from build123d import *

# Parameters (mm, degrees)
F0_R     = 12.5
F0_R_2   = 10
F1_DEPTH = 6
F0_R_3   = 2.2
F2_DEPTH = 11
F3_R     = 1.5
F4_DEPTH = 11
F5_DEPTH = 3


with BuildPart() as f1:
    # F0 (on Front) → F1 (new body)
    with BuildSketch(Plane.XZ):
        Circle(F0_R)
        Circle(F0_R_2, mode=Mode.SUBTRACT)
    extrude(amount=F1_DEPTH)

    # F0 (on Front) → F2 (join)
    with BuildSketch(Plane.XZ):
        Circle(F0_R_2)
        Circle(F0_R_3, mode=Mode.SUBTRACT)
    extrude(amount=F2_DEPTH)

    # F3 (on Front) → F4 (cut)
    with BuildSketch(Plane.XZ):
        with Locations((6.3, 0)):
            Circle(F3_R)
        with Locations((-6.3, 0)):
            Circle(F3_R)
    extrude(amount=F4_DEPTH, mode=Mode.SUBTRACT)

    # F3 (on Front) → F5 (cut)
    with BuildSketch(Plane.XZ):
        Polygon((7.970619, 2.845979), (4.670619, 2.869788), (3, 0.023809), (4.629381, -2.845979), (7.929381, -2.869788), (9.6, -0.023809), align=None)
        with Locations((6.3, 0)):
            Circle(F3_R, mode=Mode.SUBTRACT)
        Polygon((-9.6, -0.023809), (-7.929381, -2.869788), (-4.629381, -2.845979), (-3, 0.023809), (-4.670619, 2.869788), (-7.970619, 2.845979), align=None)
        with Locations((-6.3, 0)):
            Circle(F3_R, mode=Mode.SUBTRACT)
    extrude(amount=F5_DEPTH, mode=Mode.SUBTRACT)


solid = f1.part
Input: part model. Units: mm. Frame: model coordinates. A direction names the side the tool comes from. Give positions to 0.01 mm unless a question says otherwise; leave off trailing zeros. Loops run counter-clockwise (first coordinate to the right, second up) from the corner with the lowest first, then second, coordinate; pieces in that order, holes last. Notation, with made-up numbers: (60.5, 58.25) -> (110.5, 58.25) arc R12 ccw to (110.5, 68.25) -> close; hole circle Ø11 at (30, -26). An arc over 180 degrees is marked (long way). Answer as a JSON object with one key per item and string values. Group by question number.
Item 1: Cut plane D-D, the plane x = 9. Return the cut outline in (y, z).
Item 2: Line query: probe 1 along Z at (x, y) = (0, -6.5); probe 2 along Z at (x, y) = (0, -4.5); probe 3 along X at (y, z) = (-8.75, -0.25). Output: solid intervals per line, ascending.
Item 3: Reachability of faces 4 (the flat face through (-2.4, -11, 0.1)), 5 (the flat face through (8.797, -1.479, 1.391)) from +Z, -Z, +X, -X, +Y, -Y: full face, straight path, thin tool, end or side. Return the list, or none.
Item 4: Cut plane C-C, the plane z = -5.75. Return the cut outline in (x, y), and give its area (3 significant figures).
Item 5: Cut plane A-A, the plane x = 0. Return the cut outline in (y, z).
Item 6: Pull-direction query (X, two-part tool) for faces 1 (the flat face through (-0.1, -6, 10.2)), 2 (the cylindrical face through (11.923, -2.958, 3.755)), 3 (the cylindrical face through (-4.87, -6.94, 0.45)); classes: released by +X, released by -X, zero draft, split by the parting line, or undercut.
Item 7: Cut plane B-B, the plane y = -5. Return the cut outline in (x, z).
Item 8: Pin query (flat end, axial travel): P1, Ø1.5, axis at y = -3.5, z = 4.5, coming from the -X side; P2, Ø2, axis at x = 2.5, y = -8.5, coming from the +Z side; P3, Ø4, axis at y = -9, z = -3.5, coming from the +X side. Return the tip coordinate at first contact, or that it passes through.
Checks:
{
 "1": {"outline": "(-11, -4.36) -> (-6, -4.36) -> (-6, -8.67) -> (0, -8.67) -> (0, -1.05) -> (-3, -1.05) -> (-3, 1.03) -> (0, 1.03) -> (0, 8.67) -> (-6, 8.67) -> (-6, 4.36) -> (-11, 4.36) -> close"},
 "2": {"probe 1": "z = -10 to -2.2, 2.2 to 10", "probe 2": "z = -12.5 to -2.2, 2.2 to 12.5", "probe 3": "x = -10 to -7.78, -4.82 to -2.19, 2.19 to 4.82, 7.78 to 10"},
 "3": {"face 4": "+Z, -Z, +X, -X, -Y", "face 5": "+Y"},
 "4": {"outline": "(-11.1, -6) -> (-8.18, -6) -> (-8.18, -11) -> (8.18, -11) -> (8.18, -6) -> (11.1, -6) -> (11.1, 0) -> (-11.1, 0) -> close", "area": "215 mm²"},
 "5": {"outline": "(-11, -10) -> (-6, -10) -> (-6, -12.5) -> (0, -12.5) -> (0, -2.2) -> (-11, -2.2) -> close; (-11, 2.2) -> (0, 2.2) -> (0, 12.5) -> (-6, 12.5) -> (-6, 10) -> (-11, 10) -> close"},
 "6": {"face 1": "zero draft", "face 2": "split by the parting line", "face 3": "undercut"},
 "7": {"outline": "circle Ø25 at (0, 0); hole circle Ø3 at (-6.3, 0); hole circle Ø4.4 at (0, 0); hole circle Ø3 at (6.3, 0)"},
 "8": {"P1": "stops at x = -11.92", "P2": "stops at z = 9.89", "P3": "stops at x = 9.89"}
}
